Autodesk Fusion 360 part; units mm, degrees
sketch "スケッチ1" plane through (0, 0, 0) normal (0, 0, 1) x (1, 0, 0)
  line L0 (-35, -15) -> (0, -15)
  circle A0 centre (0, 0) radius 15
  line L1 (12.2873, 8.6036) -> (0.8064, 25)
  circle A1 centre (0, 0) radius 10.5
  line L2 (-29, 10.25) -> (-8, 10.25)
  line L3 (-8, 10.25) -> (-8, -10.25)
  line L4 (-8, -10.25) -> (-29, -10.25)
  line L5 (-29, -10.25) -> (-29, 10.25)
  line L6 (-13, 35) -> (13, 35)
  line L7 (-35, -15) -> (-40, -10)
  line L8 (-40, -10) -> (-40, 10)
  line L9 (-23, 15) -> (-35, 15)
  line L10 (-35, 15) -> (-40, 10)
  line L11 (0.8064, 25) -> (0.8064, 31)
  line L12 (0.8064, 31) -> (18, 31)
  line L13 (18, 31) -> (18, 39)
  line L14 (18, 39) -> (-18, 39)
  line L15 (-18, 39) -> (-23, 34)
  line L16 (-23, 34) -> (-23, 15)
  line L17 (-35, 7) -> (-7.8262, 7)
  line L18 (-7.8262, 7) -> (-7.8262, -7)
  line L19 (-7.8262, -7) -> (-35, -7)
  line L20 (-35, -7) -> (-35, 7)
  point P0 (-8, 0)
  point P1 (-11.5, 0)
  point P2 (-29.7, 0)
  point P3 (18, 35)
  point P4 (-7.8262, 0)
  dimension "d1" = 30
  dimension "d2" = 55
  dimension "d3" = 35
  dimension "d6" = 21
  dimension "d7" = 8
  dimension "d8" = 21
  dimension "d9" = 20.5
  dimension "d28" = 26
  dimension "d35" = 5
  dimension "d36" = 5
  dimension "d64" = 25
  dimension "d65" = 6
  dimension "d66" = 8
  dimension "d67" = 18
  dimension "d68" = 5
  dimension "d71" = 5
  dimension "d72" = 5
  dimension "d74" = 5
  dimension "d75" = 5
  dimension "d76" = 5
  dimension "d82" = 35
  dimension "d83" = 20
  dimension "d84" = 14
extrude "押し出し1" add sketch "スケッチ1" along normal blind 4 contours L0 A0 L1 L2 L4 L5 L7 L8 L9 L10 L11 L12 L13 L14 L15 L16 L17 L19 L20 | A0 A1 L2 L3 L4 L17 L19 | A0 L4 L5 L19 | A0 L3 L4 L19 | A0 L2 L3 L17 | A0 L2 L5 L17
hole "穴1" at (-8, 10.25, 0) at (-8, -10.25, 0) at (-29, -10.25, 0) at (-29, 10.25, 0) direction (0, 0, 1) diameter 2.1 depth 10 tip angle 118
hole "穴3" at (-13, 35, 0) at (13, 35, 0) direction (0, 0, 1) diameter 3.2 depth 10 tip angle 118
fillet "フィレット4" radius 1 10 edges at (-35, -15, 2) (-40, -10, 2) (-40, 10, 2) (-35, 15, 2) (-23, 34, 2) (-18, 39, 2) (18, 39, 2) (18, 31, 2) (0.8064, 25, 2) (0.8064, 31, 2)
fillet "フィレット5" radius 5 1 edges at (-23, 15, 2)
Part model, mm, in its own coordinate system. A direction names the side the tool comes from. Coordinates: 2 decimals unless noted, no trailing zeros. Loops run counter-clockwise (first coordinate to the right, second up) from the corner with the lowest first, then second, coordinate; pieces in that order, holes last. Notation, with made-up numbers: (2.25, 42.5) - (8.25, 42.5) arc R8 cw to (8.25, 48.5) - close; hole circle Ø11 at (-21, 80.5). An arc over 180 degrees is marked (long way). Write item = value, one per line. Start each with the question number.
Item 1: Mould opens along Y. For faces 6 (the flat face through (-37, 13, 2)), 7 (the cylindrical face through (-14.08, 33.82, 2.03)), 8 (the flat face through (-11, 12, 0)) say: released by +Y, released by -Y, zero draft, split by the parting line, or undercut.
Item 2: 3-axis set-ups, long thin cutter, end or side, ignore diameter. For faces 1 (the flat face through (-21, -7, 2)), 2 (the flat face through (-31, 15, 2)), 3 (the flat face through (-11, 12, 4)), 4 (the flat face through (6.716, 16.56, 1.972)), 5 (the flat face through (-40, 0, 2)): which of +Z, -Z, +X, -X, +Y, -Y reach the whole face in a straight line?
Item 3: Cut at D-D, the plane y = 35. Give the cut face in (x, z), and give its area (3 significant figures).
Item 4: Flat gauge pins, fed straight in: pin 1 Ø1 at (x, z) = (-26.5, 0.5) entering from +Y; pin 2 Ø1.2 at (y, z) = (28.5, 2.5) entering from -X; pin 3 Ø1.2 at (y, z) = (2.5, 2) entering from +X. Where does each tip first touch, or does it go through?
Item 5: Cut at A-A, the plane x = -21. Give the cut face in (y, z), and give its area (3 significant figures).
Item 6: Cut at B-B, the plane y = 0. Give the cut face in (x, z).
Item 7: Cut at C-C, the plane x = 13. Give the cut face in (y, z), and give its area (3 significant figures).
Item 8: Wall check: L1, parallel to Y at x = -29, z = 1.25; L2, parallel to Y at x = -13, z = 2.55; L3, parallel to Y at x = -8, z = 3. Give the ranges that are in metal, low to high. Write a range as from..to.
The answers:
q1.face_6 = released by +Y
q1.face_7 = undercut
q1.face_8 = zero draft
q2.face_1 = +Z, -Z
q2.face_2 = +Z, -Z, -X, +Y
q2.face_3 = +Z, +X, -X, +Y, -Y
q2.face_4 = +Z, -Z, +X
q2.face_5 = +Z, -Z, -X, +Y, -Y
q3.outline = (-22, 0) - (-14.6, 0) - (-14.6, 4) - (-22, 4) - close; (-11.4, 0) - (11.4, 0) - (11.4, 4) - (-11.4, 4) - close; (14.6, 0) - (18, 0) - (18, 4) - (14.6, 4) - close
q3.area = 134 mm2
q4.pin_1 = 15.42
q4.pin_2 = -23
q4.pin_3 = 14.88
q5.outline = (-15, 0) - (-7, 0) - (-7, 4) - (-15, 4) - close; (7, 0) - (36, 0) - (36, 4) - (7, 4) - close
q5.area = 148 mm2
q6.outline = (-40, 0) - (-35, 0) - (-35, 4) - (-40, 4) - close; (10.5, 0) - (15, 0) - (15, 4) - (10.5, 4) - close
q7.outline = (-7.48, 0) - (7.48, 0) - (7.48, 4) - (-7.48, 4) - close; (31, 0) - (33.4, 0) - (33.4, 4) - (31, 4) - close; (36.6, 0) - (39, 0) - (39, 4) - (36.6, 4) - close
q7.area = 79.1 mm2
q8.L1 = -15..-11.3, -9.2..-7, 7..9.2, 11.3..15
q8.L2 = -15..-7, 7..33.4, 36.6..39
q8.L3 = -15..-11.3, -9.2..-7, 7..9.2, 11.3..39
